from build123d import *

# Parameters (mm, degrees)
CHAMFER1_SIZE = 0.508


with BuildPart() as part:
    # Sketch1 → Revolve1 (revolve)
    with BuildSketch(Plane.XY):
        Polygon((-4.7625, 60.2234), (-4.7625, 57.1754), (-4.4577, 57.1754), (-4.4577, 56.4388), (-4.7625, 56.4388), (-4.7625, 24.2951), (-4.4577, 24.2951), (-4.4577, 23.5585), (-4.7625, 23.5585), (-4.7625, 7.3025), (-4.4577, 7.3025), (-4.4577, 6.5659), (-4.7625, 6.5659), (-4.7625, -6.5659), (-4.4577, -6.5659), (-4.4577, -7.3025), (-4.7625, -7.3025), (-4.7625, -23.5585), (-4.4577, -23.5585), (-4.4577, -24.2951), (-4.7625, -24.2951), (-4.7625, -56.4388), (-4.4577, -56.4388), (-4.4577, -57.1754), (-4.7625, -57.1754), (-4.7625, -60.2234), (-4.4577, -60.2234), (-4.4577, -60.96), (-4.7625, -60.96), (-4.7625, -62.23), (0, -62.23), (0, 62.23), (-4.7625, 62.23), (-4.7625, 60.96), (-4.4577, 60.96), (-4.4577, 60.2234), align=None)
    revolve(axis=Axis((0, 62.23, 0), (0, -1, 0)))

    # Chamfer1
    chamfer1_edges = [part.edges().sort_by_distance(p)[0] for p in [
        (4.7625, 62.23, 0),
        (4.7625, -62.23, 0),
    ]]
    chamfer(chamfer1_edges, length=CHAMFER1_SIZE)


solid = part.part
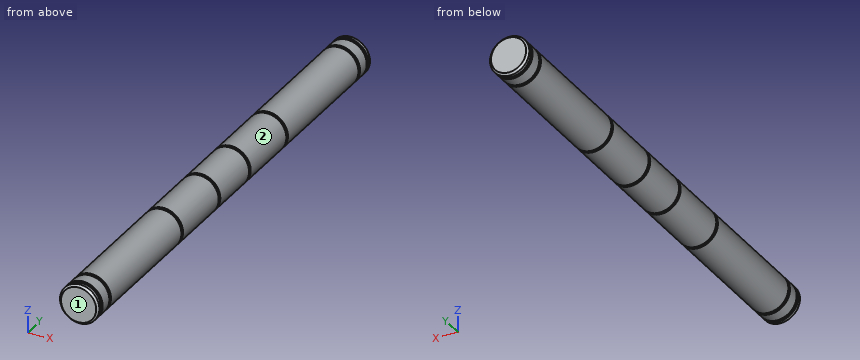
Read the model definition and answer for the solid it produces. Units are mm, in the model's axes. Face numbers are marked on the shaded views. Round coordinates to 2 decimals unless told otherwise and drop trailing zeros. Order: outer loops, then holes, each group sorted by start corner. A loop starts at its lowest first (then second) coordinate and runs counter-clockwise, first axis right, second up. Notation, with made-up numbers: (44, -30.75) - (83, -30.75) arc R30 cw to (83, 7.25) - close; hole circle Ø10 at (75.25, 67). An arc over 180 degrees is marked (long way). Use one line per item in the form item = value. Start each with the question number.
(1) The part is cut by section A-A (y = 17). Give the vertices of the cut face in (x, z) (1 decimal), then the cut area to 3 significant figures.
(2) Flat-ended cylindrical pins translate along their axes: pin 1 Ø1.5 at (x, y) = (-1, -8) entering from +Z; pin 2 Ø4 at (x, y) = (2.5, 30) entering from +Z. Find the tip coordinate at first contact, or state that the pin passes through.
(3) Determine the mould class of the marked faces 1 and 2 for opening direction X: +X half, -X half, draft (parallel to the pull), parting line (faces both ways), or undercut.
(4) Find the intervals of material crossed by line 1 along Z through (x, y) = (-1.5, -44.5); line 2 along X through (y, z) = (-44, -2.25); line 3 along Z through (x, y) = (-0.5, 14.5), in increasing order. Write a range as from..to.
Checked values:
q1.outline = circle Ø9.5 at (0, 0)
q1.area = 71.3 mm^2
q2.pin_1 = 4.76
q2.pin_2 = 4.74
q3.face_1 = draft
q3.face_2 = parting line
q4.line_1 = -4.52..4.52
q4.line_2 = -4.2..4.2
q4.line_3 = -4.74..4.74
